```python
from build123d import *

# Parameters (mm, degrees)
F0_W        = 82
F0_H        = 20
F1_DEPTH    = 30
F2_T1_DEPTH = 30
F2_T3_DEPTH = 88.7163597955
F2_T5_DEPTH = 86.5103060247
F3_R        = 5
F4_R        = 2


# Not quite as in the source:
# - a fillet or chamfer that OpenCascade refuses, or shapes differently, is made with other operations: its cross-section is extruded or revolved along the edge and cut away or added


with BuildPart() as f1:
    # F0 (on Top) → F1 (new body)
    with BuildSketch(Plane.XY):
        Polygon((-31.3680246472, 15.4572909642), (-38.791685015, 15.4572909642), (-38.791685015, -15.5427090358), (38.208314985, -15.5427090358), (38.208314985, 15.4572909642), (31.6319753528, 15.4572909642), (28.6463200748, 15.4572909642), (-28.3536799252, 15.4572909642), align=None)
        with BuildLine():
            Line((-35.617634356, 1.409011777), (-35.617634356, 12.5002924819))
            Line((-35.617634356, 12.5002924819), (-24.2628612362, 12.5002924819))
            ThreePointArc((-24.2628612362, 12.5002924819), (-23.1469813734, 12.55), (-22.0311015107, 12.5002924819))
            Line((-22.0311015107, 12.5002924819), (21.7593006052, 12.5002924819))
            ThreePointArc((21.7593006052, 12.5002924819), (22.875180468, 12.55), (23.9910603307, 12.5002924819))
            Line((23.9910603307, 12.5002924819), (35.382365644, 12.5002924819))
            Line((35.382365644, 12.5002924819), (35.382365644, 1.035769749))
            ThreePointArc((35.382365644, 1.035769749), (35.4144721936, 0.5183271366), (35.425180468, 0))
            ThreePointArc((35.425180468, 0), (35.4144721936, -0.5183271366), (35.382365644, -1.035769749))
            Line((35.382365644, -1.035769749), (35.382365644, -12.4997075181))
            Line((35.382365644, -12.4997075181), (23.9975939216, -12.4997075181))
            ThreePointArc((23.9975939216, -12.4997075181), (22.875180468, -12.55), (21.7527670144, -12.4997075181))
            Line((21.7527670144, -12.4997075181), (-22.0245679198, -12.4997075181))
            ThreePointArc((-22.0245679198, -12.4997075181), (-23.1469813734, -12.55), (-24.269394827, -12.4997075181))
            Line((-24.269394827, -12.4997075181), (-35.617634356, -12.4997075181))
            Line((-35.617634356, -12.4997075181), (-35.617634356, -1.409011777))
            ThreePointArc((-35.617634356, -1.409011777), (-35.6969813734, 0), (-35.617634356, 1.409011777))
        make_face(mode=Mode.SUBTRACT)
        Polygon((38.208314985, -15.5427090358), (-38.791685015, -15.5427090358), (-44.0882174298, -15.5427090358), (-44.0882174298, -40.5095070601), (43.0414974689, -40.5095070601), (43.0414974689, -15.5427090358), align=None)
        with Locations((-0.4833955318, -28.0716251582)):
            Rectangle(F0_W, F0_H, mode=Mode.SUBTRACT)
        Polygon((-31.3680246472, 43.4572909642), (-31.3680246472, 15.4572909642), (-28.3536799252, 15.4572909642), (-28.3536799252, 38.9038845897), (-28.3536799252, 40.4572909642), (-14.6007314324, 40.4572909642), (14.6007314324, 40.4572909642), (28.6463200748, 40.4572909642), (28.6463200748, 38.9038845897), (28.6463200748, 15.4572909642), (31.6319753528, 15.4572909642), (31.6319753528, 43.4572909642), align=None)
        with BuildLine():
            Line((35.382365644, 12.5002924819), (23.9910603307, 12.5002924819))
            ThreePointArc((23.9910603307, 12.5002924819), (31.7777528847, 8.8457167242), (35.382365644, 1.035769749))
            Line((35.382365644, 1.035769749), (35.382365644, 12.5002924819))
        make_face()
        with BuildLine():
            ThreePointArc((35.382365644, -1.035769749), (31.7800643524, -8.8433897915), (23.9975939216, -12.4997075181))
            Line((23.9975939216, -12.4997075181), (35.382365644, -12.4997075181))
            Line((35.382365644, -12.4997075181), (35.382365644, -1.035769749))
        make_face()
        with BuildLine():
            Line((-24.2628612362, 12.5002924819), (-35.617634356, 12.5002924819))
            Line((-35.617634356, 12.5002924819), (-35.617634356, 1.409011777))
            ThreePointArc((-35.617634356, 1.409011777), (-31.9163938742, 8.9777449503), (-24.2628612362, 12.5002924819))
        make_face()
        with BuildLine():
            ThreePointArc((-24.269394827, -12.4997075181), (-31.9187398511, -8.9754528136), (-35.617634356, -1.409011777))
            Line((-35.617634356, -1.409011777), (-35.617634356, -12.4997075181))
            Line((-35.617634356, -12.4997075181), (-24.269394827, -12.4997075181))
        make_face()
        Polygon((14.6007314324, 40.4572909642), (28.6463200748, 38.9038845897), (28.6463200748, 40.4572909642), align=None)
        Polygon((-28.3536799252, 40.4572909642), (-28.3536799252, 38.9038845897), (-14.6007314324, 40.4572909642), align=None)
    extrude(amount=F1_DEPTH)

    # F2: fillet of radius 13 on 4 edges, made by hand

    # F2_s2 → F2_t1 (join)
    with BuildSketch(Plane.XY):
        with BuildLine():
            ThreePointArc((-38.791685015, -5.0710049164), (-40.1911445403, -10.9384967738), (-44.0882174298, -15.5427090358))
            Line((-44.0882174298, -15.5427090358), (-38.791685015, -15.5427090358))
            Line((-38.791685015, -15.5427090358), (-38.791685015, -5.0710049164))
        make_face()
        with BuildLine():
            ThreePointArc((43.0414974689, -15.5427090358), (39.4786809816, -11.0331797269), (38.208314985, -5.4282099548))
            Line((38.208314985, -5.4282099548), (38.208314985, -15.5427090358))
            Line((38.208314985, -15.5427090358), (43.0414974689, -15.5427090358))
        make_face()
    extrude(amount=F2_T1_DEPTH)

    # F2_s4 → F2_t3 (cut)
    with BuildSketch(Plane.XY.offset(-29.3581798978)):
        with BuildLine():
            ThreePointArc((-38.791685015, 3.7140190051), (-36.7801429418, 10.6605139767), (-31.3680246472, 15.4572909642))
            Line((-31.3680246472, 15.4572909642), (-38.791685015, 15.4572909642))
            Line((-38.791685015, 15.4572909642), (-38.791685015, 3.7140190051))
        make_face()
    extrude(amount=F2_T3_DEPTH, mode=Mode.SUBTRACT)

    # F2_s6 → F2_t5 (cut)
    with BuildSketch(Plane.XY.offset(-28.2551530123)):
        with BuildLine():
            ThreePointArc((38.208314985, 4.1552297593), (36.44458627, 10.6932881568), (31.6319753528, 15.4572909642))
            Line((31.6319753528, 15.4572909642), (38.208314985, 15.4572909642))
            Line((38.208314985, 15.4572909642), (38.208314985, 4.1552297593))
        make_face()
    extrude(amount=F2_T5_DEPTH, mode=Mode.SUBTRACT)

    # F3
    f3_edges = [f1.edges().sort_by_distance(p)[0] for p in [
        (31.631975, 43.457291, 15),
        (-31.368025, 43.457291, 15),
    ]]
    fillet(f3_edges, radius=F3_R)

    # F4
    f4_edges = [f1.edges().sort_by_distance(p)[0] for p in [
        (-44.088217, -15.542709, 15),
        (-44.088217, -40.509507, 15),
        (43.041497, -40.509507, 15),
        (43.041497, -15.542709, 15),
    ]]
    fillet(f4_edges, radius=F4_R)


solid = f1.part
```
Part model, mm, in its own coordinate system. A direction names the side the tool comes from. Coordinates: 2 decimals unless noted, no trailing zeros. Write each loop counter-clockwise with the first axis right and the second up, starting at its lowest first coordinate (ties: lowest second). Pieces come first, ordered by that corner, then holes.
Item 1: Slice it at A-A (y = 33). Write the cut outline in (x, z), and give its area (3 significant figures).
Item 2: Slice it at C-C (z = 17.25). Count the separate pieces of the cut face and the enclosed holes in it, and give its area (3 significant figures).
Item 3: Slice it at D-D (y = 11). Write the cut outline in (x, z), and give its area (3 significant figures).
Item 4: Probe line 1 (Y direction, x = 14, z = 4.5); line 2 (X direction, y = 33.5, z = 27); line 3 (Y direction, x = -26, z = 6.5). List the from-to ranges inside material, lowest first.
Item 5: Slice it at B-B (x = 8.5). Write the cut outline in (y, z).
Item 6: Mould opens along X. For faces 4 (the face through (43.041, -28, 15)), 5 (the face through (-21.57, 39.67, 14.79)), 6 (the face through (-1, -14, 0)) say: released by +X, released by -X, zero draft, split by the parting line, or undercut.
Item 7: Which spindle directions (+Z, -Z, +X, -X, +Y, -Y) get a long thin tool onto all of the face, cutting with end or side? Do faces 1 (the face through (38.208, -1, 15)), 2 (the face through (-38.792, -1, 15)), 3 (the face through (1, 15.457, 15)). Say none if no direction does.
Item 8: Pin check, flat tips, straight feed: pin 1 (11.5 mm diameter, centred on y = 29.5, z = 12.5, fed in from -X); pin 2 (11.5 mm diameter, centred on y = 29.5, z = 17.5, fed in from +X); pin 3 (7.5 mm diameter, centred on y = 1.5, z = 14, fed in from +X); pin 4 (12 mm diameter, centred on x = 33, y = 21, fed in from -Z). Stop position of each tip, or through.
Results found:
1. outline: (-31.37, 0) - (-28.35, 0) - (-28.35, 30) - (-31.37, 30) - close; (28.65, 0) - (31.63, 0) - (31.63, 30) - (28.65, 30) - close
1. area: 180 mm2
2. separate pieces: 1
2. enclosed holes: 3
2. area: 1,610 mm2
3. outline: (-36.56, 0) - (-29.19, 0) - (-29.19, 30) - (-36.56, 30) - close; (28.92, 0) - (36.26, 0) - (36.26, 30) - (28.92, 30) - close
3. area: 441 mm2
4. line 1: y = -40.51 to -38.07, -18.07 to -12.5, 12.5 to 15.46, 40.46 to 43.46
4. line 2: x = -31.37 to -28.35, 28.65 to 31.63
4. line 3: y = -40.51 to -38.07, -18.07 to -12.22, 12.22 to 15.46, 39.17 to 43.46
5. outline: (-40.51, 0) - (-38.07, 0) - (-38.07, 30) - (-40.51, 30) - close; (-18.07, 0) - (-12.5, 0) - (-12.5, 30) - (-18.07, 30) - close; (12.5, 0) - (15.46, 0) - (15.46, 30) - (12.5, 30) - close; (40.46, 0) - (43.46, 0) - (43.46, 30) - (40.46, 30) - close
6. face 4: released by +X
6. face 5: undercut
6. face 6: zero draft
7. face 1: +Z, -Z, +X, +Y
7. face 2: +Z, -Z, -X, +Y
7. face 3: +Z, -Z
8. pin 1: stops at x = -31.37
8. pin 2: stops at x = 31.63
8. pin 3: stops at x = 38.21
8. pin 4: stops at z = 0
